```python
from build123d import *

# Parameters (mm, degrees)
BASPROSKE_W         = 7
BASPROSKE_H         = 13.5
TOOTHCUT_DEPTH      = 21.334699408
TEETHCUTS_COUNT     = 25
TEETHCUTS_ANGLE     = 345.6
BORSKE_R            = 0.4
BORE_DEPTH          = 50.0000508
SKETCH_1_R          = 3
SKETCH_1_R_2        = 1.65
CUT_EXTRUDE_1_DEPTH = 10
SKETCH_2_W          = 30
SKETCH_2_H          = 10
SKETCH_2_R          = 1.65
EXTRUDE_2_DEPTH     = 5
CUT_EXTRUDE_2_DEPTH = 2.5


with BuildPart() as part:
    # BasProSke → Base-Revolve (revolve)
    with BuildSketch(Plane(origin=(0, 0, 0), x_dir=(1, 0, 0), z_dir=(0, 1, 0)), mode=Mode.PRIVATE) as base_revolve_sk:
        with Locations((3.5, 6.75)):
            Rectangle(BASPROSKE_W, BASPROSKE_H)
    revolve(base_revolve_sk.sketch.rotate(Axis((-10, 0, 0), (1, 0, 0)), 180), axis=Axis((-10, 0, 0), (1, 0, 0)))

    # TooCutSke → ToothCut (cut, through all)
    with BuildSketch(Plane(origin=(0, 0, 0), x_dir=(0, 0, -1), z_dir=(1, 0, 0))):
        with BuildLine():
            ThreePointArc((0.480087995, 11.238750665), (0, 11.249), (-0.480087995, 11.238750665))
            ThreePointArc((-0.480087995, 11.238750665), (-0.821124963, 12.40220054), (-1.432168974, 13.449361962))
            ThreePointArc((-1.432168974, 13.449361962), (0, 13.5254), (1.432168974, 13.449361962))
            ThreePointArc((1.432168974, 13.449361962), (0.821124963, 12.40220054), (0.480087995, 11.238750665))
        make_face()
    toothcut = extrude(amount=TOOTHCUT_DEPTH, mode=Mode.SUBTRACT)

    # TeethCuts: ToothCut ×25 about axis
    teethcuts_axis = Axis((-10, 0, 0), (1, 0, 0))
    for i in range(1, TEETHCUTS_COUNT):
        add(toothcut.rotate(teethcuts_axis, i * TEETHCUTS_ANGLE / (TEETHCUTS_COUNT - 1)), mode=Mode.SUBTRACT)

    # BorSke → Bore (cut, symmetric)
    with BuildSketch(Plane(origin=(0, 0, 0), x_dir=(0, 0, -1), z_dir=(1, 0, 0))):
        with Locations(Location((0, 0, 0), (0, 0, 180))):
            Circle(BORSKE_R)
    extrude(amount=BORE_DEPTH, both=True, mode=Mode.SUBTRACT)

    # 草图1 → 切除-拉伸1 (cut)
    with BuildSketch(Plane(origin=(7, 0, 0), x_dir=(0, 0, -1), z_dir=(1, 0, 0))):
        Circle(SKETCH_1_R)
        with Locations((0, 7)):
            Circle(SKETCH_1_R_2)
        with Locations((7, 0)):
            Circle(SKETCH_1_R_2)
        with Locations((-7, 0)):
            Circle(SKETCH_1_R_2)
        with Locations((0, -7)):
            Circle(SKETCH_1_R_2)
    extrude(amount=-CUT_EXTRUDE_1_DEPTH, mode=Mode.SUBTRACT)

    # 草图2 → 凸台-拉伸2 (add)
    with BuildSketch(Plane(origin=(7, 0, 0), x_dir=(0, 0, -1), z_dir=(1, 0, 0))):
        with Locations((-24, 0)):
            Rectangle(SKETCH_2_W, SKETCH_2_H)
        with Locations((-31, 0)):
            Circle(SKETCH_2_R, mode=Mode.SUBTRACT)
        with Locations((-19, 0)):
            Circle(SKETCH_2_R, mode=Mode.SUBTRACT)
    extrude(amount=-EXTRUDE_2_DEPTH)

    # 草图3 → 切除-拉伸2 (cut)
    with BuildSketch(Plane(origin=(7, 0, 0), x_dir=(0, 0, -1), z_dir=(1, 0, 0))):
        Polygon((-15.651368439, 0), (-17.325684219, 2.9), (-20.674315781, 2.9), (-22.348631561, 0), (-20.674315781, -2.9), (-17.325684219, -2.9), align=None)
        Polygon((-27.651368439, 0), (-29.325684219, 2.9), (-32.674315781, 2.9), (-34.348631561, 0), (-32.674315781, -2.9), (-29.325684219, -2.9), align=None)
    extrude(amount=-CUT_EXTRUDE_2_DEPTH, mode=Mode.SUBTRACT)


solid = part.part
```
Here's how the part is built. I have some questions about the finished solid (model axes, mm). A direction names the side the tool comes from. Coordinates: 2 decimals unless noted, no trailing zeros. Loops run counter-clockwise (first coordinate to the right, second up) from the corner with the lowest first, then second, coordinate; pieces in that order, holes last. Notation, with made-up numbers: (36.25, 38.25) - (61.25, 38.25) arc R18 ccw to (61.25, 48.25) - close; hole circle Ø10 at (23.25, 54.5). An arc over 180 degrees is marked (long way). Return JSON: item names as keys, results as strings. Group by question number.
Item 1: If we section it at D-D on z = 21.5: Write out the boundary of the cut face in (x, y), and give its area (3 significant figures).
Item 2: I need wall thicknesses on line 1 (Y direction, x = 3.25, z = 0); line 2 (Z direction, x = 6.5, y = 0.5); line 3 (Y direction, x = 3.5, z = 17). Which ranges of each line are inside material? Lowest first, please. Write a range as from..to.
Item 3: If we section it at B-B on y = 7: Write out the boundary of the cut face in (x, z), and give its area (3 significant figures).
Item 4: If we section it at C-C on x = 6.5: State how many separate pieces and enclosed holes the cut face has, and give its area (3 significant figures).
Item 5: Will these pins go through, and if not, where does the flat tip stop? P1, Ø3, axis at x = 5.5, z = 19.5, coming from the +Y side; P2, Ø3, axis at y = 0, z = 19, coming from the +X side; P3, Ø10, axis at y = 8, z = 17, coming from the -X side; P4, Ø0.8, axis at x = 5.5, z = 32, coming from the -Y side.
Item 6: If we section it at A-A on z = 31: Write out the boundary of the cut face in (x, y), and give its area (4 significant figures).
Item 7: We'd pull the mould along Y, two halves only. Please class faces 4 (the face through (3.45, -10.49, 6.62)), 5 (the face through (3.45, -12.17, -2.35)), 6 (the face through (3.45, 3.05, -12.05)): +Y half, -Y half, draft (parallel to the pull), parting line (faces both ways), or undercut.
Item 8: On a 3-axis mill with a long thin cutter (end or side, diameter ignored), from which of +Z, -Z, +X, -X, +Y, -Y can I reach the whole of each face in a straight line? I mean faces 1 (the face through (3.45, 7.34, 10.03)), 2 (the face through (3.451, -12.377, 0.748)), 3 (the face through (0.986, 0.713, 11.226)). Say none if no direction works.
Calculated:
{
 "1": {"outline": "(2, -5) - (7, -5) - (7, -1.47) - (4.5, -1.47) - (4.5, 1.47) - (7, 1.47) - (7, 5) - (2, 5) - close", "area": "42.7 mm^2"},
 "2": {"line 1": "y = -13.5..-8.65, -5.35..-3, 3..5.35, 8.65..11.25", "line 2": "z = -11.24..-8.57, -5.43..-2.96, 2.96..5.43, 8.57..15.94, 22.06..27.94, 34.06..39", "line 3": "y = -5..5"},
 "3": {"outline": "(0, -9.78) - (7, -9.78) - (7, -1.65) - (0, -1.65) - close; (0, 1.65) - (7, 1.65) - (7, 9.78) - (0, 9.78) - close", "area": "114 mm^2"},
 "4": {"separate pieces": "1", "enclosed holes": "7", "area": "627 mm^2"},
 "5": {"P1": "stops at y = 5", "P2": "passes through", "P3": "stops at x = 2", "P4": "stops at y = -5"},
 "6": {"outline": "(2, -5) - (7, -5) - (7, -2.9) - (4.5, -2.9) - (4.5, -1.65) - (2, -1.65) - close; (2, 1.65) - (4.5, 1.65) - (4.5, 2.9) - (7, 2.9) - (7, 5) - (2, 5) - close", "area": "27.25 mm^2"},
 "7": {"face 4": "undercut", "face 5": "-Y half", "face 6": "undercut"},
 "8": {"face 1": "+Z, +X, -X", "face 2": "+X, -X, -Y", "face 3": "+Z, -X"}
}
